Design review of the part built by this model. Coordinates are the model's own, in mm. Coordinates: 2 decimals unless noted, no trailing zeros. Loops run counter-clockwise (first coordinate to the right, second up) from the corner with the lowest first, then second, coordinate; pieces in that order, holes last. Notation, with made-up numbers: M 79,38 L 125,38 A31 cw 125,75 Z; hole C 33,-16 d2. An arc over 180 degrees is marked long. Answer as a JSON object with one key per item and string values. Group by question number.
1. Consider section B-B (y = 0.7). State the section outline as (x, z) points.
2. Consider section C-C (z = 0). State the section outline as (x, y) points, then the cut area to 3 significant figures.
3. Insertion check: pin 1 (1.5 mm diameter, centred on x = -13, y = 1, fed in from +Z); pin 2 (0.9 mm diameter, centred on y = 2, z = 48.5, fed in from -X). Each pin has a flat end and moves straight along its axis. Give the tip position at first contact, or say it passes through.
4. Consider section D-D (z = 44). State the section outline as (x, y) points.
5. To check wall thickness, follow probe 1 along Z at (x, y) = (30.5, 2.25); probe 2 along X at (y, z) = (1.3, 12.5); probe 3 along X at (y, z) = (0.2, 2). State the ranges of each line that lie inside material, in increasing order.
6. Consider section A-A (x = 26). State the section outline as (y, z) points.
from build123d import *

# Parameters (mm, degrees)
SKETCH2_W           = 4
SKETCH2_H           = 60
BOSS_EXTRUDE1_DEPTH = 3


with BuildPart() as part:
    # Sketch2 → Boss-Extrude1 (new body)
    # profile 1 of 2: a face of its own
    with BuildSketch(Plane(origin=(0, 0, 0), x_dir=(1, 0, 0), z_dir=(0, 1, 0))):
        with BuildLine():
            Line((-32, 5), (32, 5))
            ThreePointArc((32, 5), (37, 0), (32, -5))
            Line((32, -5), (-32, -5))
            ThreePointArc((-32, -5), (-37, 0), (-32, 5))
        make_face()
        with BuildLine():
            ThreePointArc((32, -3), (35, 0), (32, 3))
            Line((32, 3), (-32, 3))
            ThreePointArc((-32, 3), (-35, 0), (-32, -3))
            Line((-32, -3), (32, -3))
        make_face(mode=Mode.SUBTRACT)
    # profile 2 of 2: a face of its own
    with BuildSketch(Plane(origin=(0, 0, 0), x_dir=(1, 0, 0), z_dir=(0, 1, 0))):
        with Locations((0, -35)):
            Rectangle(SKETCH2_W, SKETCH2_H)
    extrude(amount=BOSS_EXTRUDE1_DEPTH)


solid = part.part
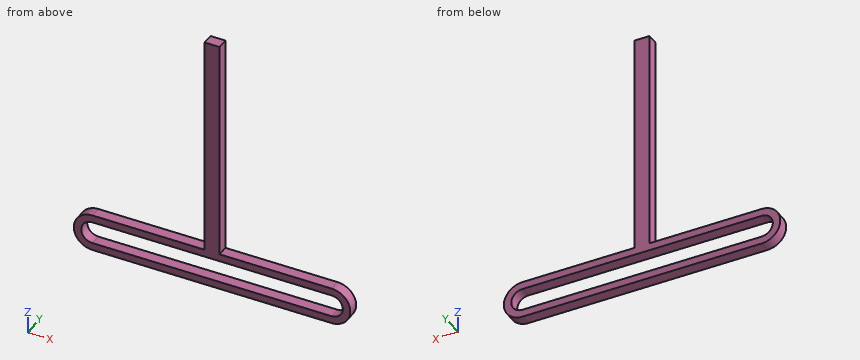
Findings below:
{
 "1": {"outline": "M -32,-5 L 32,-5 A5 ccw 32,5 L 2,5 L 2,65 L -2,65 L -2,5 L -32,5 A5 ccw Z; hole M -32,-3 L 32,-3 A3 ccw 32,3 L -32,3 A3 ccw Z"},
 "2": {"outline": "M -37,0 L -35,0 L -35,3 L -37,3 Z; M 35,0 L 37,0 L 37,3 L 35,3 Z", "area": "12.0 mm^2"},
 "3": {"pin 1": "stops at z = 5", "pin 2": "stops at x = -2"},
 "4": {"outline": "M -2,0 L 2,0 L 2,3 L -2,3 Z"},
 "5": {"probe 1": "z = -5 to -3, 3 to 5", "probe 2": "x = -2 to 2", "probe 3": "x = -36.58 to -34.24, 34.24 to 36.58"},
 "6": {"outline": "M 0,-5 L 3,-5 L 3,-3 L 0,-3 Z; M 0,3 L 3,3 L 3,5 L 0,5 Z"}
}
